Autodesk Inventor part; units mm, degrees
ref_plane "YZ Plane" through (0, 0, 0) normal (1, 0, 0) x (0, 1, 0)
ref_plane "XZ Plane" through (0, 0, 0) normal (0, 1, 0) x (-1, 0, 0)
ref_plane "XY Plane" through (0, 0, 0) normal (0, 0, 1) x (1, 0, 0)
sketch "Sketch1" plane through (0, 0, 0) normal (0, 1, 0) x (-1, 0, 0)
  line L0 (180.5524, 781.9255) -> (180.551, 788.2755)
  line L1 (180.551, 788.2755) -> (174.551, 788.2742)
  line L2 (174.551, 788.2742) -> (174.5524, 781.9242)
  line L3 (174.5524, 781.9242) -> (168.4524, 781.9229)
  line L4 (168.4524, 781.9229) -> (168.4537, 775.9228)
  line L5 (168.4537, 775.9228) -> (169.7037, 775.9231)
  line L6 (169.7037, 775.9231) -> (169.7042, 773.9231)
  line L7 (169.7042, 773.9231) -> (168.4542, 773.9229)
  line L8 (168.4542, 773.9229) -> (168.4547, 771.2728)
  line L9 (168.4547, 771.2728) -> (165.4547, 771.2722)
  line L10 (165.4547, 771.2722) -> (165.4541, 773.9222)
  line L11 (165.4541, 773.9222) -> (164.2041, 773.9219)
  line L12 (164.2041, 773.9219) -> (164.2037, 775.9219)
  line L13 (164.2037, 775.9219) -> (165.4537, 775.9222)
  line L14 (165.4537, 775.9222) -> (165.4524, 781.9222)
  line L15 (165.4524, 781.9222) -> (159.3524, 781.9209)
  line L16 (159.3524, 781.9209) -> (159.351, 788.2709)
  line L17 (159.351, 788.2709) -> (153.351, 788.2696)
  line L18 (153.351, 788.2696) -> (153.3524, 781.9196)
  line L19 (153.3524, 781.9196) -> (141.9524, 781.9171)
  line L20 (141.9524, 781.9171) -> (153.9094, 749.9197)
  line L21 (153.9094, 749.9197) -> (153.9122, 737.1696)
  line L22 (153.9122, 737.1696) -> (148.9122, 737.1685)
  line L23 (148.9122, 737.1685) -> (148.9139, 729.3686)
  line L24 (148.9139, 729.3686) -> (153.9139, 729.3697)
  line L25 (153.9139, 729.3697) -> (154.0889, 729.3947)
  line L26 (154.0889, 729.3947) -> (155.1888, 729.545)
  line L27 (155.1888, 729.545) -> (156.4138, 730.0452)
  line L28 (156.4138, 730.0452) -> (157.4386, 730.8204)
  line L29 (157.4386, 730.8204) -> (158.2386, 731.8705)
  line L30 (158.2386, 731.8705) -> (189.9642, 775.495)
  line L31 (189.9642, 775.495) -> (189.9628, 781.9276)
  line L32 (189.9628, 781.9276) -> (180.5524, 781.9255)
  point P0 (0, 0)
extrude "Extrusion1" add sketch "Sketch1" along normal blind 6
properties part number "Z Motor Mount Brace_CPY"
Design review of the part built by this model. Coordinates are the model's own, in mm. A direction names the side the tool comes from. Coordinates: 2 decimals unless noted, no trailing zeros. Loops run counter-clockwise (first coordinate to the right, second up) from the corner with the lowest first, then second, coordinate; pieces in that order, holes last.
Q1. We need section C-C on x = -152.5. State the section outline as (y, z) points.
Reported:
outline: (0, 729.37) - (6, 729.37) - (6, 737.17) - (0, 737.17) - close; (0, 753.69) - (6, 753.69) - (6, 781.92) - (0, 781.92) - close
Q2. We need section D-D on z = 745.5. State the section outline as (x, y) points.
Reported:
outline: (-168.15, 0) - (-153.91, 0) - (-153.91, 6) - (-168.15, 6) - close
Q3. Tool access review of faces 1 (the face through (-147.85, 2.96, 766.14)), 2 (the face through (-166, 6, 766)): name each direction out of +Z, -Z, +X, -X, +Y, -Y from which nothing blocks a thin tool from reaching the whole face with its end or side.
Reported:
face 1: +X, +Y, -Y
face 2: +Z, -Z, +X, -X, +Y
Q4. For pin 1 (3 mm diameter, centred on y = 3.5, z = 784, fed in from +X); pin 2 (1 mm diameter, centred on x = -169, y = 4, fed in from -Z); pin 3 (1.8 mm diameter, centred on y = 2.5, z = 785.5, fed in from -X), all flat-tipped, find the tip position at first contact; note any pin that passes through.
Reported:
pin 1: stops at x = -153.35
pin 2: stops at z = 745.98
pin 3: stops at x = -180.55
Q5. To check wall thickness, follow line 1 (X direction, y = 1.5, z = 784.5); line 2 (X direction, y = 3.75, z = 776.5); line 3 (X direction, y = 1, z = 749). State the ranges of each line that lie inside material, in increasing order.
Reported:
line 1: x = -180.55 to -174.55, -159.35 to -153.35
line 2: x = -189.96 to -168.45, -165.45 to -143.98
line 3: x = -170.7 to -153.91
Q6. We need section B-B on z = 783. State the section outline as (x, y) points, and give its area (3 significant figures).
Reported:
outline: (-180.55, 0) - (-174.55, 0) - (-174.55, 6) - (-180.55, 6) - close; (-159.35, 0) - (-153.35, 0) - (-153.35, 6) - (-159.35, 6) - close
area: 72.0 mm2
